```python
from build123d import *

# Parameters (mm, degrees)
SKETCH1_R                  = 15
SKETCH1_R_2                = 4
BOSS_EXTRUDE1_DEPTH        = 14
M4X0_7_TAPPED_HOLE1_REACH  = 36.371
M4X0_7_TAPPED_HOLE1_BORE_R = 1.65
M4X0_7_TAPPED_HOLE3_D      = 3.3
M4X0_7_TAPPED_HOLE3_DEPTH  = 8
M4X0_7_TAPPED_HOLE3_TIP    = 0.991420021


with BuildPart() as part:
    # Sketch1 → Boss-Extrude1 (new body)
    with BuildSketch(Plane.XY):
        Circle(SKETCH1_R)
        Circle(SKETCH1_R_2, mode=Mode.SUBTRACT)
    extrude(amount=BOSS_EXTRUDE1_DEPTH)

    # M4x0.7 Tapped Hole1 bore (on position points) → M4x0.7 Tapped Hole1 (cut, up to next)
    with BuildSketch(Plane(origin=(0.246830438, 14.99796902, 7), x_dir=(0.999864601356, -0.016455362532, 0), z_dir=(0.016455362532, 0.999864601356, 0)), mode=Mode.PRIVATE) as m4x0_7_tapped_hole1_sk1:
        Circle(M4X0_7_TAPPED_HOLE1_BORE_R)
    m4x0_7_tapped_hole1_tool1 = extrude(m4x0_7_tapped_hole1_sk1.sketch, amount=-M4X0_7_TAPPED_HOLE1_REACH, mode=Mode.PRIVATE) & part.part
    add(m4x0_7_tapped_hole1_tool1.solids().sort_by_distance((0.24683, 14.997969, 7))[0], mode=Mode.SUBTRACT)

    # M4x0.7 Tapped Hole3
    with Locations(Plane(origin=(0, 0, 0), x_dir=(-1, 0, 0), z_dir=(0, 0, -1))):
        with Locations((0, 12), (-12, 0), (0, -12), (12, 0)):
            Hole(M4X0_7_TAPPED_HOLE3_D / 2, depth=M4X0_7_TAPPED_HOLE3_DEPTH)
            with Locations((0, 0, -(M4X0_7_TAPPED_HOLE3_DEPTH + M4X0_7_TAPPED_HOLE3_TIP / 2))):  # 118° drill point
                Cone(0, M4X0_7_TAPPED_HOLE3_D / 2, M4X0_7_TAPPED_HOLE3_TIP, mode=Mode.SUBTRACT)


solid = part.part
```
The listing builds one solid part. Answer for the finished solid, in the listing's coordinates (mm). A direction names the side the tool comes from. Give positions to 0.01 mm unless a question says otherwise; leave off trailing zeros. Write each loop counter-clockwise with the first axis right and the second up, starting at its lowest first coordinate (ties: lowest second). Pieces come first, ordered by that corner, then holes. Notation, with made-up numbers: M 10.5,13 L 27.5,13 A33 cw 27.5,47 Z; hole C 51.25,24 d1. An arc over 180 degrees is marked long. Write each question's results on one line, items separated by ' | '.
Q1. Section A-A, the plane y = 2.5 is taken. Write down the section's boundary in (x, z), then the cut area to 3 significant figures.
Output values:
outline: M -14.79,0 L -3.12,0 L -3.12,14 L -14.79,14 Z; M 3.12,0 L 14.79,0 L 14.79,14 L 3.12,14 Z | area: 327 mm2
Q2. Flat-ended cylindrical pins translate along their axes: P1, Ø3, axis at x = -12, y = 0, coming from the -Z side; P2, Ø1, axis at x = -9, z = 9.5, coming from the -Y side; P3, Ø6, axis at x = -12, z = 1.5, coming from the -Y side. Find the tip coordinate at first contact, or state that the pin passes through.
Output values:
P1: z = 8.09 | P2: y = -12.36 | P3: y = -12
Q3. Section C-C, the plane y = -9 is taken. Write down the section's boundary in (x, z).
Output values:
outline: M -12,0 L 12,0 L 12,14 L -12,14 Z
Q4. Section B-B, the plane x = -3 is taken. Write down the section's boundary in (y, z).
Output values:
outline: M -14.7,0 L -2.65,0 L -2.65,14 L -14.7,14 Z; M 2.65,0 L 14.7,0 L 14.7,14 L 2.65,14 Z
Q5. Section D-D, the plane x = 6 is taken. Write down the section's boundary in (y, z).
Output values:
outline: M -13.75,0 L 13.75,0 L 13.75,14 L -13.75,14 Z
Q6. For a pull along Y with two mould halves and no side action, classify faces 1 (the cylindrical face through (-1.65, 12.07, 3.17)), 2 (the cylindrical face through (-14.985, 0.66, 6.902)), 3 (the flat face through (3, -3, 0)) as released by +Y, released by -Y, zero draft, split by the parting line, or undercut.
Output values:
face 1: undercut | face 2: split by the parting line | face 3: zero draft
Q7. A tool of negligible diameter and unlimited length cuts with its end or side. For faces 4 (the cylindrical face through (0.92, 9.39, 8.46)), 5 (the flat face through (3, -3, 14)), 6 (the cylindrical face through (13.524, -0.632, 4.056)), from which of +Z, -Z, +X, -X, +Y, -Y can it reach the whole face along a straight path? Write none if from no direction.
Output values:
face 4: none | face 5: +Z, +X, -X, +Y, -Y | face 6: -Z
Q8. Consider L1, parallel to Y at x = 0, z = 3.25; L2, parallel to Y at x = 0, z = 5.75; L3, parallel to Y at x = -3, z = 13. Determine where each line is inside the solid, lowest interval first. Write a range as from..to.
Output values:
L1: -15..-13.65, -10.35..-4, 4..10.35, 13.65..15 | L2: -15..-13.65, -10.35..-4 | L3: -14.7..-2.65, 2.65..14.7
